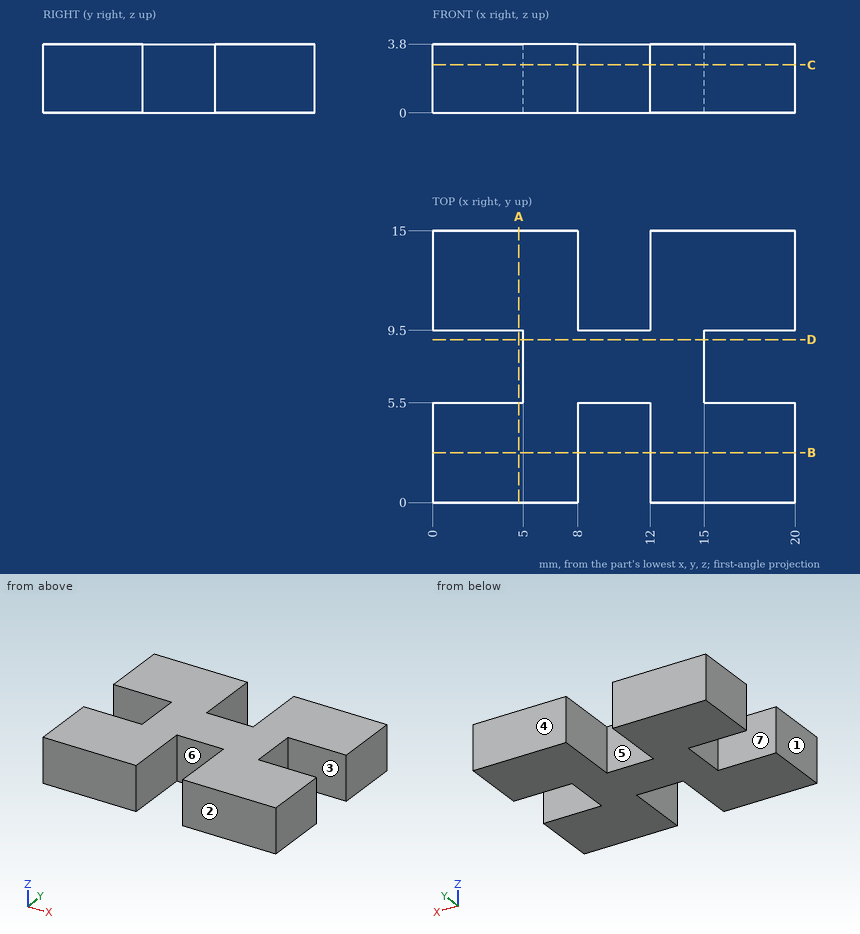
Geometry check sheet. Reference: drawing and pictorial views, mm from the part's lowest x, y, z. A direction names the side the tool comes from. Give positions to 0.01 mm unless a question says otherwise; leave off trailing zeros. Write each loop counter-clockwise with the first axis right and the second up, starting at its lowest first coordinate (ties: lowest second). Pieces come first, ordered by that corner, then holes. Notation, with made-up numbers: M -13,62 L 32,62 A12 cw 32,84 Z; hole C 75,12.25 d8. An arc over 180 degrees is marked long. Put each result on its own line as item: value. Start each with the question number.
1. Section check B-B (y = 2.75). Record the cut outline in (x, z).
2. Go/stop test with flat-tipped pins: pin 1 Ø1.1 at (x, z) = (2.5, 2.5) entering from -Y; pin 2 Ø1.1 at (y, z) = (7.5, 3) entering from +X. Record where each tip stops, or that it passes through.
3. Set-up check for the marked faces 5, 6 and 7: record each of +Z, -Z, +X, -X, +Y, -Y from which the full face is reachable in a straight line by a thin tool's end or side.
4. Section check C-C (z = 2.65). Record the cut outline in (x, y).
5. Section check A-A (x = 4.75). Record the cut outline in (y, z), and give its area (3 significant figures).
6. Scan lines: line 1 along X through (y, z) = (1.5, 3.4); line 2 along Y through (x, z) = (17.25, 2.85); line 3 along X through (y, z) = (7.5, 0.2). Record each from-to range of solid material in increasing order. Write a range as [from, to].
7. Draft check along Y on the marked faces 1, 2, 3 and 4. Enter one of: +Y half, -Y half, draft (parallel to the pull), parting line (faces both ways), or undercut.
8. Section check D-D (y = 9). Record the cut outline in (x, z), and give its area (3 significant figures).
Answer list:
1. outline: M 0,0 L 8,0 L 8,3.8 L 0,3.8 Z; M 12,0 L 20,0 L 20,3.8 L 12,3.8 Z
2. pin 1: y = 0
2. pin 2: x = 15
3. face 5: +Z, -Z, +Y
3. face 6: +Z, -Z, -Y
3. face 7: +Z, -Z, -X
4. outline: M 0,0 L 8,0 L 8,5.5 L 12,5.5 L 12,0 L 20,0 L 20,5.5 L 15,5.5 L 15,9.5 L 20,9.5 L 20,15 L 12,15 L 12,9.5 L 8,9.5 L 8,15 L 0,15 L 0,9.5 L 5,9.5 L 5,5.5 L 0,5.5 Z
5. outline: M 0,0 L 5.5,0 L 5.5,3.8 L 0,3.8 Z; M 9.5,0 L 15,0 L 15,3.8 L 9.5,3.8 Z
5. area: 41.8 mm2
6. line 1: [0, 8], [12, 20]
6. line 2: [0, 5.5], [9.5, 15]
6. line 3: [5, 15]
7. face 1: draft
7. face 2: -Y half
7. face 3: undercut
7. face 4: +Y half
8. outline: M 5,0 L 15,0 L 15,3.8 L 5,3.8 Z
8. area: 38.0 mm2
